from build123d import *

# Parameters (mm, degrees)
SKETCH1_R           = 38.1
BOSS_EXTRUDE1_DEPTH = 76.2
SHELL2_T            = 3.175
SCALE1_SCALE        = 0.615384615


with BuildPart() as part:
    # Sketch1 → Boss-Extrude1 (new body)
    with BuildSketch(Plane(origin=(0, 0, 0), x_dir=(1, 0, 0), z_dir=(0, 1, 0))):
        with Locations(Location((0, 0, 0), (0, 0, 90))):
            Circle(SKETCH1_R)
    extrude(amount=BOSS_EXTRUDE1_DEPTH)

    # Shell2
    shell2_openings = [part.faces().sort_by_distance(p)[0] for p in [
        (0, 76.2, 0),
    ]]
    offset(amount=SHELL2_T, openings=shell2_openings, kind=Kind.INTERSECTION)


with BuildPart() as part_1:
    # Scale1: scaled about (0, 29.378039662, 0)
    add(part.part.scale(SCALE1_SCALE).moved(Location((0, 11.299246024, 0))))


solid = part_1.part
Can you work these out from the model? Positions are in its coordinate system, mm. A direction names the side the tool comes from. Give positions to 0.01 mm unless a question says otherwise; leave off trailing zeros. Order: outer loops, then holes, each group sorted by start corner. A loop starts at its lowest first (then second) coordinate and runs counter-clockwise, first axis right, second up. Notation, with made-up numbers: M 6,82.25 L 61,82.25 A24 ccw 61,119.25 Z; hole C 81.25,54.5 d4. An arc over 180 degrees is marked long. Use one line per item in the form item = value. Start each with the question number.
Item 1: If we section it at B-B (x = 0): Write out the boundary of the cut face in (y, z), then the cut area to 3 significant figures.
Item 2: If we section it at C-C (y = 15): Write out the boundary of the cut face in (x, z).
Item 3: Will these pins go through, and if not, where does the flat tip stop? pin 1 Ø1 at (x, y) = (-1.5, 27) entering from -Z; pin 2 Ø2 at (y, z) = (22, -13.5) entering from +X; pin 3 Ø5 at (y, z) = (16.5, 14) entering from -X.
Item 4: We'd pull the mould along Z, two halves only. Please class faces 1 (the flat face through (0, 11.299, 0)), 2 (the cylindrical face through (15.456, 33.427, 20.157)), 3 (the flat face through (22.5, 58.192, -7.4)): +Z half, -Z half, draft (parallel to the pull), parting line (faces both ways), or undercut.
Item 5: If I drill on line 1 along X through (y, z) = (45, 0); line 2 along Z through (x, y) = (-2, 21.5); line 3 along Y through (x, z) = (2, -8), over which ranges is the centre line in solid material (lowest first)?
Item 6: For faces 4 (the cylindrical face through (22.89, 34.42, 5.08)), 5 (the flat face through (0, 9.345, 0)), which set-ups out of +Z, -Z, +X, -X, +Y, -Y let a thin tool reach every point of the face, with its end or its side?
Item 7: If we section it at A-A (z = 0): Write out the boundary of the cut face in (x, y), then the cut area to 3 significant figures.
Outcome:
q1.outline = M 9.35,-25.4 L 58.19,-25.4 L 58.19,-23.45 L 11.3,-23.45 L 11.3,23.45 L 58.19,23.45 L 58.19,25.4 L 9.35,25.4 Z
q1.area = 282 mm2
q2.outline = C 0,0 d50.8; hole C 0,0 d46.89
q3.pin_1 = -25.38
q3.pin_2 = 22.11
q3.pin_3 = -22.65
q4.face_1 = undercut
q4.face_2 = parting line
q4.face_3 = draft
q5.line_1 = -25.4 to -23.45, 23.45 to 25.4
q5.line_2 = -25.32 to -23.36, 23.36 to 25.32
q5.line_3 = 9.35 to 11.3
q6.face_4 = +Y
q6.face_5 = +Z, -Z, +X, -X, -Y
q7.outline = M -25.4,9.35 L 25.4,9.35 L 25.4,58.19 L 23.45,58.19 L 23.45,11.3 L -23.45,11.3 L -23.45,58.19 L -25.4,58.19 Z
q7.area = 282 mm2
